Could you check a few things on this model? Use its own coordinates, in mm. Face numbers are marked on the shaded views. A direction names the side the tool comes from. Give positions to 0.01 mm unless a question says otherwise; leave off trailing zeros. Order: outer loops, then holes, each group sorted by start corner. A loop starts at its lowest first (then second) coordinate and runs counter-clockwise, first axis right, second up. Notation, with made-up numbers: (31.5, -29.5) -> (90.5, -29.5) arc R14 cw to (90.5, -2.5) -> close; hole circle Ø11 at (14, -10). An arc over 180 degrees is marked (long way). One line per item, written item: value.
```python
from build123d import *

# Parameters (mm, degrees)
AUFSATZ_LINEAR_AUSTRAGEN1_DEPTH = 10
SKIZZE2_R                       = 1.75
SCHNITT_LINEAR_AUSTRAGEN1_DEPTH = 64.625859523
SKIZZE4_R                       = 2.2
SCHNITT_LINEAR_AUSTRAGEN3_DEPTH = 74.305456823
VERRUNDUNG1_R                   = 10


with BuildPart() as part:
    # Skizze1 → Aufsatz-Linear austragen1 (new body)
    with BuildSketch(Plane.XY):
        with BuildLine():
            Line((0.5, -28.495613698), (0.5, -32.496153619))
            Line((0.5, -32.496153619), (0.5, -38.496153619))
            Line((0.5, -38.496153619), (3.5, -38.496153619))
            Line((3.5, -38.496153619), (3.5, -32.310988843))
            ThreePointArc((3.5, -32.310988843), (31.468752272, -8.122045953), (18.7, 26.581196361))
            Line((18.7, 26.581196361), (18.7, 51.5))
            Line((18.7, 51.5), (10.2, 51.5))
            Line((10.2, 51.5), (10.2, 31.5))
            Line((10.2, 31.5), (-10.2, 31.5))
            Line((-10.2, 31.5), (-10.2, 51.5))
            Line((-10.2, 51.5), (-18.7, 51.5))
            Line((-18.7, 51.5), (-18.7, 26.581196361))
            ThreePointArc((-18.7, 26.581196361), (-31.468752272, -8.122045953), (-3.5, -32.310988843))
            Line((-3.5, -32.310988843), (-3.5, -38.496153619))
            Line((-3.5, -38.496153619), (-0.5, -38.496153619))
            Line((-0.5, -38.496153619), (-0.5, -32.496153619))
            Line((-0.5, -32.496153619), (-0.5, -28.495613698))
            ThreePointArc((-0.5, -28.495613698), (0, 28.5), (0.5, -28.495613698))
        make_face()
    extrude(amount=AUFSATZ_LINEAR_AUSTRAGEN1_DEPTH)

    # Skizze2 → Schnitt-Linear austragen1 (cut, through all)
    with BuildSketch(Plane.ZY.offset(3.5)):
        with Locations((5, -35.403571231)):
            Circle(SKIZZE2_R)
    extrude(amount=-SCHNITT_LINEAR_AUSTRAGEN1_DEPTH, mode=Mode.SUBTRACT)

    # Skizze4 → Schnitt-Linear austragen3 (cut, through all)
    with BuildSketch(Plane.ZY.offset(18.7)):
        with Locations(Location((5, 41.5, 0), (0, 0, 270))):
            Circle(SKIZZE4_R)
    extrude(amount=-SCHNITT_LINEAR_AUSTRAGEN3_DEPTH, mode=Mode.SUBTRACT)

    # Verrundung1
    verrundung1_edges = [part.edges().sort_by_distance(p)[0] for p in [
        (-18.7, 26.581196361, 5),
        (18.7, 26.581196361, 5),
    ]]
    fillet(verrundung1_edges, radius=VERRUNDUNG1_R)


solid = part.part
```
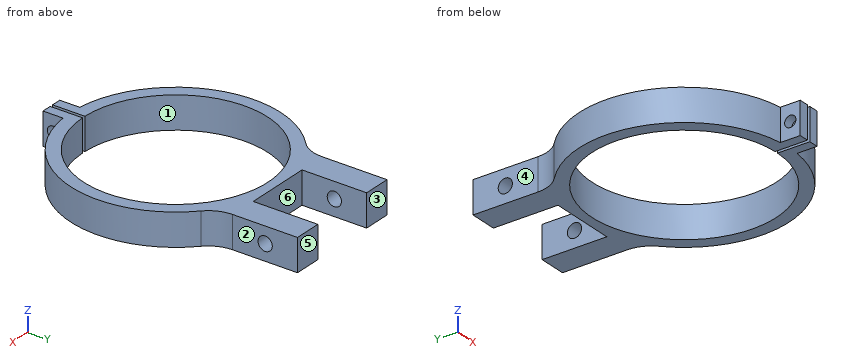
1) For P1, Ø2, axis at y = 3.5, z = 1.5, coming from the +X side; P2, Ø4.5, axis at y = -35.4, z = 5, coming from the -X side; P3, Ø1.9, axis at y = -35, z = 2.5, coming from the +X side, each with a flat end and sliding along its axis, tell me the tip position at first contact or that it passes through.
Answer below:
P1: stops at x = 32.4
P2: stops at x = -3.5
P3: stops at x = 3.5
2) For the marked faces 4, 5 and 6, which set-ups out of +Z, -Z, +X, -X, +Y, -Y let a thin tool reach every point of the face, with its end or its side?
Answer below:
face 4: +Z, -Z, -X, +Y
face 5: +Z, -Z, +X, -X, +Y
face 6: +Z, -Z, +Y
3) We'd pull the mould along Y, two halves only. Please class the marked faces 1, 2 and 3: +Y half, -Y half, draft (parallel to the pull), parting line (faces both ways), or undercut.
Answer below:
face 1: undercut
face 2: draft
face 3: +Y half
4) Suppose I cut it at A-A, the plane x = 13. Write out the boundary of the cut face in (y, z).
Answer below:
outline: (-29.79, 0) -> (-25.36, 0) -> (-25.36, 10) -> (-29.79, 10) -> close; (25.36, 0) -> (51.5, 0) -> (51.5, 10) -> (25.36, 10) -> close; hole circle Ø4.4 at (41.5, 5)
5) Suppose I cut it at D-D, the plane y = 41.5. Write out the boundary of the cut face in (x, z).
Answer below:
outline: (-18.7, 0) -> (-10.2, 0) -> (-10.2, 2.8) -> (-18.7, 2.8) -> close; (-18.7, 7.2) -> (-10.2, 7.2) -> (-10.2, 10) -> (-18.7, 10) -> close; (10.2, 0) -> (18.7, 0) -> (18.7, 2.8) -> (10.2, 2.8) -> close; (10.2, 7.2) -> (18.7, 7.2) -> (18.7, 10) -> (10.2, 10) -> close
6) Suppose I cut it at B-B, the plane z = 5. State how many separate pieces and enclosed holes the cut face has, then the cut area to 3 significant figures.
Answer below:
separate pieces: 5
enclosed holes: 0
area: 1,080 mm2
7) Suppose I cut it at C-C, the plane y = 0. Write out the boundary of the cut face in (x, z).
Answer below:
outline: (-32.5, 0) -> (-28.5, 0) -> (-28.5, 10) -> (-32.5, 10) -> close; (28.5, 0) -> (32.5, 0) -> (32.5, 10) -> (28.5, 10) -> close
8) If I drill on line 1 along X through (y, z) = (47.5, 3.75); line 2 along Y through (x, z) = (2.7, 5); line 3 along X through (y, z) = (0, 6), over which ranges is the centre line in solid material (lowest first)?
Answer below:
line 1: x = -18.7 to -10.2, 10.2 to 18.7
line 2: y = -38.5 to -37.15, -33.65 to -28.37, 28.37 to 31.5
line 3: x = -32.5 to -28.5, 28.5 to 32.5
